The listing builds one solid part. Answer for the finished solid, in the listing's coordinates (mm). A direction names the side the tool comes from. Round coordinates to 2 decimals unless told otherwise and drop trailing zeros. Write each loop counter-clockwise with the first axis right and the second up, starting at its lowest first coordinate (ties: lowest second). Pieces come first, ordered by that corner, then holes. Notation, with made-up numbers: (-37.75, -34.5) - (-33.75, -34.5) arc R9 cw to (-33.75, -19.5) - close; hole circle Ø1 at (80, 23.25). An arc over 180 degrees is marked (long way). Use a Markdown table: item, result. Add a question column.
1) Each of these flat-tipped pins is pushed along its axis until it touches: P1, Ø10, axis at x = 8.5, z = 68, coming from the +Y side; P2, Ø3.5, axis at x = -17.5, y = 0, coming from the -Z side. Where does it stop, or does it pass through?
2) Find the intervals of material crossed by probe 1 along X at (y, z) = (0, 9); probe 2 along X at (y, z) = (-2.25, 35.55); probe 3 along Z at (x, y) = (-4, -2.5), in increasing order. Write a range as from..to.
3) A cutting plane is placed at A-A (z = 8.75). Give the vertices of the cut face in (x, y), then the cut area to 3 significant figures.
4) A cutting plane is placed at C-C (x = -9). Give the vertices of the cut face in (y, z), then the cut area to 3 significant figures.
5) A tool of negligible diameter and unlimited length cuts with its end or side. For faces 4 (the flat face through (0, 2, 43.55)), 5 (the cylindrical face through (-15.497, 0.631, 7.301)), 6 (the flat face through (0, -3, 0)), from which of +Z, -Z, +X, -X, +Y, -Y can it reach the whole face along a straight path? Write none if from no direction.
6) A cutting plane is placed at D-D (z = 83.5). Give the vertices of the cut face in (x, y).
7) Determine the mould class of faces 1 (the cylindrical face through (15.773, -0.089, 102.368)), 2 (the cylindrical face through (2.003, 0.631, 7.301)), 3 (the flat face through (0, -6.35, 54)) for opening direction Y: +Y half, -Y half, draft (parallel to the pull), parting line (faces both ways), or undercut.
8) A cutting plane is placed at B-B (y = -4.75). Give the vertices of the cut face in (x, z).
```python
from build123d import *

# Parameters (mm, degrees)
SKETCH12_W                = 50
SKETCH12_H                = 12.7
BOSS_EXTRUDE1_DEPTH       = 110
M5X0_8_TAPPED_HOLE2_D     = 4.2
M5X0_8_TAPPED_HOLE2_DEPTH = 14.4
M5X0_8_TAPPED_HOLE2_TIP   = 1.2618073
M5X0_8_TAPPED_HOLE3_D     = 4.2
SKETCH23_R                = 2.55
CUT_EXTRUDE2_DEPTH        = 114.517795962
SKETCH26_W                = 34
SKETCH26_H                = 52.9
CUT_EXTRUDE1_DEPTH        = 9.7
FILLET1_R                 = 5


with BuildPart() as part:
    # Sketch12 → Boss-Extrude1 (new body)
    with BuildSketch(Plane.XY):
        Rectangle(SKETCH12_W, SKETCH12_H)
    extrude(amount=BOSS_EXTRUDE1_DEPTH)

    # M5x0.8 Tapped Hole2
    with Locations(Plane(origin=(0, 0, 0), x_dir=(-1, 0, 0), z_dir=(0, 0, -1))):
        with Locations((-17.5, 0), (0, 0), (17.5, 0)):
            Hole(M5X0_8_TAPPED_HOLE2_D / 2, depth=M5X0_8_TAPPED_HOLE2_DEPTH)
            with Locations((0, 0, -(M5X0_8_TAPPED_HOLE2_DEPTH + M5X0_8_TAPPED_HOLE2_TIP / 2))):  # 118° drill point
                Cone(0, M5X0_8_TAPPED_HOLE2_D / 2, M5X0_8_TAPPED_HOLE2_TIP, mode=Mode.SUBTRACT)

    # M5x0.8 Tapped Hole3 (through all)
    with Locations(Plane(origin=(0, 6.35, 0), x_dir=(1, 0, 0), z_dir=(0, 1, 0))):
        with Locations((-0.5, -35.55), (15.5, -35.55), (15.5, -104.45), (-0.5, -104.45)):
            Hole(M5X0_8_TAPPED_HOLE3_D / 2)

    # Sketch23 → Cut-Extrude2 (cut, through all)
    with BuildSketch(Plane.XZ.offset(6.35)):
        with Locations(Location((-9, 8.75, 0), (0, 0, 270))):
            Circle(SKETCH23_R)
        with Locations(Location((9, 8.75, 0), (0, 0, 270))):
            Circle(SKETCH23_R)
    extrude(amount=-CUT_EXTRUDE2_DEPTH, mode=Mode.SUBTRACT)

    # Sketch26 → Cut-Extrude1 (cut)
    with BuildSketch(Plane(origin=(0, 6.35, 0), x_dir=(1, 0, 0), z_dir=(0, 1, 0))):
        with Locations((0, -70)):
            Rectangle(SKETCH26_W, SKETCH26_H)
    extrude(amount=-CUT_EXTRUDE1_DEPTH, mode=Mode.SUBTRACT)

    # Fillet1
    fillet1_edges = [part.edges().sort_by_distance(p)[0] for p in [
        (-25, 0, 110),
        (25, 0, 110),
        (-17, 1.5, 96.45),
        (-17, 1.5, 43.55),
        (17, 1.5, 43.55),
        (17, 1.5, 96.45),
    ]]
    fillet(fillet1_edges, radius=FILLET1_R)


solid = part.part
```
Entries:
| question | item | result |
|---|---|---|
| 1 | P1 | stops at y = -3.35 |
| 1 | P2 | stops at z = 14.61 |
| 2 | probe 1 | x = -25..-19.6, -15.4..-11.54, -6.46..-2.1, 2.1..6.46, 11.54..15.4, 19.6..25 |
| 2 | probe 2 | x = -25..-2.6, 1.6..13.4, 17.6..25 |
| 2 | probe 3 | z = 0..43.55, 96.45..110 |
| 3 | outline | (-25, -6.35) - (-11.55, -6.35) - (-11.55, 6.35) - (-25, 6.35) - close; (-6.45, -6.35) - (6.45, -6.35) - (6.45, 6.35) - (-6.45, 6.35) - close; (11.55, -6.35) - (25, -6.35) - (25, 6.35) - (11.55, 6.35) - close; hole circle Ø4.2 at (-17.5, 0); hole circle Ø4.2 at (0, 0); hole circle Ø4.2 at (17.5, 0) |
| 3 | area | 464 mm² |
| 4 | outline | (-6.35, 0) - (6.35, 0) - (6.35, 6.2) - (-6.35, 6.2) - close; (-6.35, 11.3) - (6.35, 11.3) - (6.35, 43.55) - (-3.35, 43.55) - (-3.35, 96.45) - (6.35, 96.45) - (6.35, 110) - (-6.35, 110) - close |
| 4 | area | 819 mm² |
| 5 | face 4 | +Y |
| 5 | face 5 | -Z |
| 5 | face 6 | -Z, +X, -X, +Y, -Y |
| 6 | outline | (-25, -6.35) - (25, -6.35) - (25, 6.35) - (17, 6.35) - (17, -3.35) - (-17, -3.35) - (-17, 6.35) - (-25, 6.35) - close |
| 7 | face 1 | draft |
| 7 | face 2 | undercut |
| 7 | face 3 | -Y half |
| 8 | outline | (-25, 0) - (25, 0) - (25, 105) arc R5 ccw to (20, 110) - (-20, 110) arc R5 ccw to (-25, 105) - close; hole circle Ø5.1 at (-9, 8.75); hole circle Ø4.2 at (-0.5, 35.55); hole circle Ø4.2 at (-0.5, 104.45); hole circle Ø5.1 at (9, 8.75); hole circle Ø4.2 at (15.5, 35.55); hole circle Ø4.2 at (15.5, 104.45) |
